Here's how the part is built. I have some questions about the finished solid (model axes, mm). A direction names the side the tool comes from. Round coordinates to 2 decimals unless told otherwise and drop trailing zeros. Order: outer loops, then holes, each group sorted by start corner. A loop starts at its lowest first (then second) coordinate and runs counter-clockwise, first axis right, second up.
```python
from build123d import *

# Parameters (mm, degrees)
F0_R      = 12.0113110687
F1_DEPTH  = 3.2
F2_R      = 1.5698041018
F3_DEPTH  = 25
F8_DEPTH  = 25
F11_DEPTH = 25


with BuildPart() as f1:
    # F0 (on Top) → F1 (new body)
    with BuildSketch(Plane.XY):
        Circle(F0_R)
    extrude(amount=F1_DEPTH)

    # F2 (on face) → F3 (cut)
    with BuildSketch(Plane.XY.offset(3.2)):
        Circle(F2_R)
    extrude(amount=-F3_DEPTH, mode=Mode.SUBTRACT)

    # F6 (on face) → F8 (cut)
    with BuildSketch(Plane.XY.offset(3.2)):
        with BuildLine():
            ThreePointArc((-0.7770120639, 2.3781697719), (0.0011061793, 2.5018868855), (0.7791147181, 2.3774817491))
            Line((0.7791147181, 2.3774817491), (3.2505495474, 9.9191069603))
            Line((3.2505495474, 9.9191069603), (-3.25061474, 9.9490266293))
            Line((-3.25061474, 9.9490266293), (-0.7770120639, 2.3781697719))
        make_face()
        with BuildLine():
            ThreePointArc((2.0223107656, 1.4729896057), (2.3789737797, 0.774546943), (2.50188713, 0))
            Line((2.50188713, 0), (10.4379784316, 0))
            Line((10.4379784316, 0), (8.4454240277, 6.1513897963))
            Line((8.4454240277, 6.1513897963), (2.0223107656, 1.4729896057))
        make_face()
        with BuildLine():
            ThreePointArc((2.0364204787, -1.4534203952), (1.4823509758, -2.0154589542), (0.7807718841, -2.3769380464))
            Line((0.7807718841, -2.3769380464), (3.2505495474, -9.8957903683))
            Line((3.2505495474, -9.8957903683), (8.4810052067, -6.0530062765))
            Line((8.4810052067, -6.0530062765), (2.0364204787, -1.4534203952))
        make_face()
        with BuildLine():
            Line((-3.1185087282, -9.9669527262), (-0.7470875355, -2.3877393965))
            ThreePointArc((-0.7470875355, -2.3877393965), (-1.4513145315, -2.0379218194), (-2.0121805403, -1.4867981317))
            Line((-2.0121805403, -1.4867981317), (-8.3845453337, -6.1953319237))
            Line((-8.3845453337, -6.1953319237), (-3.1185087282, -9.9669527262))
        make_face()
        with BuildLine():
            Line((-10.4126818478, 0), (-2.50188713, 0))
            ThreePointArc((-2.50188713, 0), (-2.3804302696, 0.7700590516), (-2.0278522018, 1.4653513773))
            Line((-2.0278522018, 1.4653513773), (-8.4268115461, 6.089319475))
            Line((-8.4268115461, 6.089319475), (-10.4126818478, 0))
        make_face()
    extrude(amount=-F8_DEPTH, mode=Mode.SUBTRACT)

    # F10 (on face) → F11 (cut)
    with BuildSketch(Plane(origin=(0, 0, 0), x_dir=(1, 0, 0), z_dir=(0, 0, -1))):
        with BuildLine():
            ThreePointArc((-6.2165933365, 0.5757423441), (-5.9476825457, 1.8980474954), (-5.4009304255, 3.1316868454))
            ThreePointArc((-5.4009304255, 3.1316868454), (-7.2331832359, 2.3082814558), (-6.2165933365, 0.5757423441))
        make_face()
        with BuildLine():
            ThreePointArc((-4.5983108671, 1.8980474954), (-4.8166264567, 2.6339252369), (-5.4009304255, 3.1316868454))
            ThreePointArc((-5.4009304255, 3.1316868454), (-5.9476825457, 1.8980474954), (-6.2165933365, 0.5757423441))
            ThreePointArc((-6.2165933365, 0.5757423441), (-5.0938841732, 0.8531397167), (-4.5983108671, 1.8980474954))
        make_face()
        with BuildLine():
            ThreePointArc((-1.2560993846, 6.1155315627), (0, 6.2431972545), (1.2560993846, 6.1155315627))
            ThreePointArc((1.2560993846, 6.1155315627), (1.2609516612, 6.17928246), (1.2625704704, 6.2431972545))
            ThreePointArc((1.2625704704, 6.2431972545), (-0.0639147945, 7.5041489157), (-1.2560993846, 6.1155315627))
        make_face()
        with BuildLine():
            ThreePointArc((-1.2560993846, 6.1155315627), (0, 4.9806267841), (1.2560993846, 6.1155315627))
            ThreePointArc((1.2560993846, 6.1155315627), (0, 6.2431972545), (-1.2560993846, 6.1155315627))
        make_face()
        with BuildLine():
            ThreePointArc((5.4126141971, 3.1114497445), (4.6846825015, 1.4954228894), (6.2142952239, 0.6000390224))
            ThreePointArc((6.2142952239, 0.6000390224), (5.9475248318, 1.8985416334), (5.4126141971, 3.1114497445))
        make_face()
        with BuildLine():
            ThreePointArc((5.4126141971, 3.1114497445), (5.9475248318, 1.8985416334), (6.2142952239, 0.6000390224))
            ThreePointArc((6.2142952239, 0.6000390224), (6.9748788004, 1.0607950749), (7.2731475055, 1.8985416334))
            ThreePointArc((7.2731475055, 1.8985416334), (6.6714674425, 3.0090291703), (5.4126141971, 3.1114497445))
        make_face()
        with BuildLine():
            ThreePointArc((5.0638266611, -5.0062423526), (4.971794998, -4.5194305693), (4.7084027941, -4.0998115917))
            ThreePointArc((4.7084027941, -4.0998115917), (3.730288121, -5.0062423526), (2.5819813441, -5.6842663816))
            ThreePointArc((2.5819813441, -5.6842663816), (4.0817235312, -6.2926397214), (5.0638266611, -5.0062423526))
        make_face()
        with BuildLine():
            ThreePointArc((2.5819813441, -5.6842663816), (3.730288121, -5.0062423526), (4.7084027941, -4.0998115917))
            ThreePointArc((4.7084027941, -4.0998115917), (2.9335035935, -3.9369157166), (2.5819813441, -5.6842663816))
        make_face()
        with BuildLine():
            ThreePointArc((-4.6663905471, -4.1475669037), (-3.6536564941, -5.0624407337), (-2.4663245936, -5.7353949261))
            ThreePointArc((-2.4663245936, -5.7353949261), (-2.3339839606, -5.4104188814), (-2.2888765166, -5.0624407337))
            ThreePointArc((-2.2888765166, -5.0624407337), (-3.1635211919, -3.7887092971), (-4.6663905471, -4.1475669037))
        make_face()
        with BuildLine():
            ThreePointArc((-4.6663905471, -4.1475669037), (-4.4523557862, -6.1691041097), (-2.4663245936, -5.7353949261))
            ThreePointArc((-2.4663245936, -5.7353949261), (-3.6536564941, -5.0624407337), (-4.6663905471, -4.1475669037))
        make_face()
    extrude(amount=-F11_DEPTH, mode=Mode.SUBTRACT)


solid = f1.part
```
1. On a 3-axis mill with a long thin cutter (end or side, diameter ignored), from which of +Z, -Z, +X, -X, +Y, -Y can I reach the whole of each face in a straight line? I mean faces 1 (the flat face through (0, -3, 0)), 2 (the flat face through (5.279, 3.845, 1.622)). Say none if no direction works.
Evaluation:
face 1: -Z, +X, -X, +Y, -Y
face 2: +Z, -Z
2. If we section it at C-C, the plane y = -4: Write out the boundary of the cut face in (x, z), and give its area (3 significant figures).
Evaluation:
outline: (-11.33, 0) - (-5.41, 0) - (-5.41, 3.2) - (-11.33, 3.2) - close; (-1.25, 0) - (1.31, 0) - (1.31, 3.2) - (-1.25, 3.2) - close; (5.6, 0) - (11.33, 0) - (11.33, 3.2) - (5.6, 3.2) - close
area: 45.4 mm2
3. I need wall thicknesses on probe 1 along X at (y, z) = (-2.25, 0.25); probe 2 along Y at (x, z) = (3.5, 2.6); probe 3 along X at (y, z) = (-6, 1.15). Which ranges of each line are inside material? Lowest first, please.
Evaluation:
probe 1: x = -11.8 to -7.25, -4.65 to -3.05, -1.09 to 1.09, 3.15 to 4.67, 7.23 to 11.8
probe 2: y = -11.49 to -9.71, -2.5 to 0, 2.55 to 3.69, 6.32 to 11.49
probe 3: x = -10.41 to -8.12, -1.88 to -1.24, 1.24 to 1.97, 8.41 to 10.41
4. If we section it at A-A, the plane x = 6.5: Write out the boundary of the cut face in (y, z).
Evaluation:
outline: (-10.1, 0) - (-7.51, 0) - (-7.51, 3.2) - (-10.1, 3.2) - close; (-4.64, 0) - (-3.1, 0) - (-3.1, 3.2) - (-4.64, 3.2) - close; (-0.69, 0) - (0, 0) - (0, 3.2) - (-0.69, 3.2) - close; (4.73, 0) - (10.1, 0) - (10.1, 3.2) - (4.73, 3.2) - close
5. If we section it at D-D, the plane z = 1.5: State how many separate pieces and enclosed holes the cut face has, and give its area (3 significant figures).
Evaluation:
separate pieces: 1
enclosed holes: 11
area: 267 mm2
6. If we section it at B-B, the plane x = 9.25: Write out the boundary of the cut face in (y, z), and give its area (3 significant figures).
Evaluation:
outline: (-7.66, 0) - (0, 0) - (0, 3.2) - (-7.66, 3.2) - close; (3.67, 0) - (7.66, 0) - (7.66, 3.2) - (3.67, 3.2) - close
area: 37.3 mm2
7. I'm going to push flat-ended pins straight in: P1, Ø1.5, axis at y = -8.5, z = 0.5, coming from the -X side; P2, Ø1.6, axis at x = -7.5, z = 1, coming from the +Y side; P3, Ø1.5, axis at x = -1, z = 2, coming from the +Y side. Where does each tip first touch, or does it pass through?
Evaluation:
P1: stops at x = -9.18
P2: stops at y = 9.97
P3: stops at y = 12.01
